Autodesk Inventor part; units mm, degrees
ref_plane "YZ Plane" through (0, 0, 0) normal (1, 0, 0) x (0, 1, 0)
ref_plane "XZ Plane" through (0, 0, 0) normal (0, 1, 0) x (-1, 0, 0)
ref_plane "XY Plane" through (0, 0, 0) normal (0, 0, 1) x (1, 0, 0)
sketch "Sketch1" plane through (0, 0, 0) normal (0, 0, 1) x (1, 0, 0)
  line L0 (0, -2) -> (0, -41)
  line L1 (2, -43) -> (41, -43)
  line L2 (43, -41) -> (43, -2)
  line L3 (41, 0) -> (2, 0)
  arc A0 (0, -41) -> (2, -43) centre (2, -41) ccw
  arc A1 (43, -2) -> (41, 0) centre (41, -2) ccw
  arc A2 (2, 0) -> (0, -2) centre (2, -2) ccw
  arc A3 (41, -43) -> (43, -41) centre (41, -41) ccw
  point P0 (0, 0)
  point P1 (0, -43)
  point P2 (43, -43)
  point P3 (43, 0)
  dimension "d0" = 43
  dimension "d1" = 43
  dimension "d7" = 2
extrude "Extrusion1" add sketch "Sketch1" along normal blind 50
sketch "Sketch2" plane through (0, 0, 0) normal (0, 0, -1) x (-1, 0, 0)
  line L0 (-43, -41) -> (-43, -2)
  line L1 (-2, -43) -> (-41, -43)
  line L2 (-43, 0) -> (0, -43)
  line L3 (0, -43) -> (0, 0)
  line L4 (0, 0) -> (-43, -43)
  circle A0 centre (-21.5, -21.5) radius 2.5
  circle A1 centre (-21.5, -21.5) radius 11
  dimension "d4" = 5
  dimension "d8" = 22
extrude "Extrusion2" add sketch "Sketch2" along normal blind 25 contours A0 L4 L2 | L2 L4 A0 | L4 A0 L2 | L2 A0 L4
ref_plane "Work Plane2" through (21.5, -41, 0) normal (1, 0, 0) x (0, 0, -1)
ref_plane "Work Plane3" through (21.5, -21.5, -25) normal (0, 0, -1) x (-1, 0, 0)
properties part number "motor"
Geometry: final body of the model. Coordinates: model frame, mm. A direction names the side the tool comes from. Coordinates: 2 decimals unless noted, no trailing zeros. Order: outer loops, then holes, each group sorted by start corner. A loop starts at its lowest first (then second) coordinate and runs counter-clockwise, first axis right, second up.
(1) First-contact query: pin 1 (10 mm diameter, centred on x = 37, y = -32, fed in from -Z). Flat tip, straight axial feed; report the tip coordinate or a pass-through.
(2) Access query for faces 1 (the face through (23.34, -23.19, -12.32)), 2 (the face through (0, -21, 25)). Directions: +Z, -Z, +X, -X, +Y, -Y. A direction counts if a zero-diameter tool reaches every point of the face in a straight line with its end or side. Return the directions, or none.
(3) Section query D-D (x = 3.5). Return the cut outline in (y, z), plus the area to 3 significant figures.
(4) Material intervals for probe 1 along Z at (x, y) = (4, -13.5); probe 2 along Y at (x, z) = (41.5, 17), sorted ascending.
(5) Section query A-A (y = -21.5). Return the cut outline in (x, z), plus the area to 4 significant figures.
(6) Section query C-C (z = -16.5). Return the cut outline in (x, y), plus the area to 3 significant figures.
(7) Section query B-B (x = 21.5). Return the cut outline in (y, z).
Solution:
1. pin 1: stops at z = 0
2. face 1: -Z
2. face 2: +Z, -Z, -X, +Y, -Y
3. outline: (-43, 0) - (0, 0) - (0, 50) - (-43, 50) - close
3. area: 2,150 mm2
4. probe 1: z = 0 to 50
4. probe 2: y = -42.94 to -0.06
5. outline: (0, 0) - (19, 0) - (19, -25) - (24, -25) - (24, 0) - (43, 0) - (43, 50) - (0, 50) - close
5. area: 2,275 mm2
6. outline: circle Ø5 at (21.5, -21.5)
6. area: 19.6 mm2
7. outline: (-43, 0) - (-24, 0) - (-24, -25) - (-19, -25) - (-19, 0) - (0, 0) - (0, 50) - (-43, 50) - close
